Autodesk Inventor part; units mm, degrees
ref_plane "YZ Plane" through (0, 0, 0) normal (1, 0, 0) x (0, 1, 0)
ref_plane "XZ Plane" through (0, 0, 0) normal (0, 1, 0) x (-1, 0, 0)
ref_plane "XY Plane" through (0, 0, 0) normal (0, 0, 1) x (1, 0, 0)
sketch "Sketch1" plane through (0, 0, 0) normal (0, 1, 0) x (-1, 0, 0)
  line L0 (0, 0) -> (-762, 0)
  line L1 (-762, 0) -> (-762, -914.4)
  line L2 (-762, -914.4) -> (0, -914.4)
  line L3 (0, -914.4) -> (0, 0)
  dimension "d0" = 762
  dimension "d1" = 914.4
extrude "Extrusion1" add sketch "Sketch1" along normal blind 19.05
sketch "Sketch5" plane through (762, 0, -914.4) normal (0, 0, -1) x (-1, 0, 0)
  line L0 (0, 0) -> (0, 19.05)
  line L1 (0, 0) -> (762, 0)
  line L2 (762, 0) -> (762, 19.05)
  line L3 (762, 628.65) -> (762, 781.05)
  line L4 (762, 781.05) -> (0, 609.6)
  line L5 (0, 609.6) -> (762, 609.6) construction
  line L6 (762, 19.05) -> (762, 628.65) construction
  line L7 (762, 781.05) -> (757.8183, 799.6354)
  line L8 (757.8183, 799.6354) -> (-4.1817, 628.1854)
  line L9 (0, 609.6) -> (84.6693, 628.65)
  line L10 (-4.1817, 628.1854) -> (0, 609.6)
  line L11 (0, 19.05) -> (762, 19.05)
  dimension "d22" = 152.4
  dimension "d23" = 12.68
  dimension "d25" = 19.05
  dimension "d26" = 90
  dimension "d28" = 90
  dimension "d29" = 90
extrude "Extrusion5" add sketch "Sketch5" against normal up to surface (914.4 mm away) contours L4 L10 L8 L7
sketch "Sketch7" plane through (0, 19.05, 0) normal (0, 1, 0) x (1, 0, 0)
  line L0 (0, 0) -> (762, 0)
  line L1 (0, 914.4) -> (0, 0)
  line L2 (762, 914.4) -> (0, 914.4)
  line L3 (762, 0) -> (762, 914.4)
  line L4 (762, 0) -> (762, 914.4)
  line L5 (0, 914.4) -> (0, 0)
  line L6 (762, 914.4) -> (0, 914.4)
  line L7 (0, 914.4) -> (0, 895.35)
  line L8 (0, 895.35) -> (742.95, 895.35)
  line L9 (762, 895.35) -> (762, 914.4)
  line L10 (762, 914.4) -> (742.95, 914.4)
  line L11 (742.95, 895.35) -> (742.95, 457.2)
  line L12 (742.95, 457.2) -> (762, 457.2)
  line L13 (762, 457.2) -> (762, 914.4)
  dimension "d38" = 19.05
  dimension "d39" = 19.05
  dimension "d40" = 457.2
extrude "Extrusion7" add sketch "Sketch7" along normal blind 609.6 contours L1 L2 L3 L12 L11 L8
sketch "Sketch8" plane through (762, 0, -914.4) normal (0, 0, -1) x (-1, 0, 0)
  line L0 (0, 0) -> (762, 0)
  line L1 (762, 0) -> (762, 628.65)
  line L2 (84.6667, 628.65) -> (762, 628.65)
  line L3 (84.6667, 628.65) -> (762, 781.05)
  line L4 (762, 781.05) -> (757.8183, 799.6354)
  line L5 (757.8183, 799.6354) -> (-4.1817, 628.1854)
  line L6 (-4.1817, 628.1854) -> (0, 609.6)
  line L7 (0, 0) -> (0, 609.6)
  line L8 (762, 628.65) -> (762, 781.05)
  line L9 (84.6667, 628.65) -> (762, 781.05)
  line L10 (762, 781.05) -> (84.6667, 628.65)
  line L11 (84.6667, 628.65) -> (762, 628.65)
extrude "Extrusion8" add sketch "Sketch8" against normal blind 19.05 contours L2 L3 L8
ref_plane "Work Plane2" through (762, 0, -457.2) normal (0, 0, -1) x (-1, 0, 0)
mirror "Mirror1" about plane through (762, 0, -457.2) normal (0, 0, -1) of "Extrusion7"
sketch "Sketch9" plane through (0, 0, 0) normal (0, 0, 1) x (1, 0, 0)
  line L0 (766.1817, 628.1854) -> (762, 609.6)
  line L1 (4.1817, 799.6354) -> (766.1817, 628.1854)
  line L2 (0, 781.05) -> (4.1817, 799.6354)
  line L3 (677.3333, 628.65) -> (0, 781.05)
  line L4 (677.3333, 628.65) -> (0, 628.65)
  line L5 (0, 0) -> (0, 628.65)
  line L6 (0, 0) -> (762, 0)
  line L7 (762, 0) -> (762, 609.6)
  line L8 (0, 19.05) -> (0, 781.05)
  line L9 (0, 628.65) -> (0, 781.05)
  line L10 (0, 781.05) -> (677.3333, 628.65)
  line L11 (0, 781.05) -> (742.95, 613.8863)
  line L12 (0, 628.65) -> (677.3333, 628.65)
extrude "Extrusion9" add sketch "Sketch9" against normal blind 19.05 contours L3 L4 L8
sketch "Sketch12" plane through (742.95, 19.05, -895.35) normal (-1, 0, 0) x (0, 0, 1)
  line L0 (0, 594.8363) -> (876.3, 594.8363)
  line L1 (0, 0) -> (0, 594.8363)
  line L2 (876.3, 0) -> (0, 0)
  line L3 (876.3, 0) -> (876.3, 594.8363)
  line L4 (0, 0) -> (0, 594.8363)
  line L5 (876.3, 0) -> (876.3, 762)
  line L6 (0, 442.4363) -> (876.3, 442.4363)
  line L7 (876.3, 442.4363) -> (876.3, 423.3862)
  line L8 (876.3, 423.3862) -> (0, 423.3862)
  line L9 (0, 423.3862) -> (0, 442.4363)
  point P0 (895.35, -19.05)
  dimension "d57" = 19.05
  dimension "d58" = 152.4
extrude "Extrusion10" add sketch "Sketch12" along normal up to surface (742.95 mm away) contours L6 L3 L8 L1
sketch "Sketch13" plane through (742.95, 461.4863, -19.05) normal (0, 1, 0) x (1, 0, 0)
  line L0 (-742.95, 0) -> (-742.95, 876.3)
  line L1 (0, 876.3) -> (-742.95, 876.3)
  line L2 (0, 0) -> (0, 876.3)
  line L3 (-742.95, 0) -> (0, 0)
  line L4 (0, 0) -> (0, 876.3)
  line L5 (-742.95, 876.3) -> (-742.95, 0)
  line L6 (0, 438.15) -> (-742.95, 438.15)
  line L7 (-742.95, 438.15) -> (-742.95, 419.1)
  line L8 (-742.95, 419.1) -> (0, 419.1)
  line L9 (0, 419.1) -> (0, 438.15)
  point P0 (-742.95, -19.05)
  dimension "d61" = 19.05
extrude "Extrusion11" add sketch "Sketch13" along normal up to surface contours L0 L6 L2 L8 surface through (0, 781.05, -914.4) normal (-0.2195, -0.9756, 0)
sketch "Sketch14" plane through (4.1817, 799.6354, -914.4) normal (-0.9756, 0.2195, 0) x (0, 0, 1)
  line L0 (914.4, -19.05) -> (914.4, 0)
  line L1 (0, 0) -> (914.4, 0)
  line L2 (0, -19.05) -> (0, 0)
  line L3 (0, -19.05) -> (19.05, -19.05)
  line L4 (19.05, -19.05) -> (457.2, -19.05)
  line L5 (457.2, -19.05) -> (476.25, -19.05)
  line L6 (476.25, -19.05) -> (895.35, -19.05)
  line L7 (895.35, -19.05) -> (914.4, -19.05)
  line L8 (914.4, -781.05) -> (914.4, -19.05)
  line L9 (0, 0) -> (914.4, 0)
  line L10 (914.4, 0) -> (914.4, -19.05)
  line L11 (914.4, -19.05) -> (0, -19.05)
  line L12 (0, -19.05) -> (0, 0)
extrude "Extrusion12" add sketch "Sketch14" along normal blind 127
sketch "Sketch15" plane through (742.95, 19.05, -895.35) normal (-1, 0, 0) x (0, 0, 1)
  line L0 (876.3, 423.3862) -> (0, 423.3862)
  line L1 (0, 0) -> (0, 423.3862)
  line L2 (876.3, 0) -> (0, 0)
  line L3 (876.3, 0) -> (876.3, 423.3862)
  line L4 (876.3, 423.3862) -> (0, 423.3862)
  line L5 (0, 0) -> (876.3, 0)
  line L6 (438.15, 423.3862) -> (457.2, 423.3862)
  line L7 (457.2, 423.3862) -> (457.2, 0)
  line L8 (457.2, 0) -> (438.15, 0)
  line L9 (438.15, 0) -> (438.15, 423.3862)
  point P0 (895.35, -19.05)
  dimension "d66" = 19.05
extrude "Extrusion13" add sketch "Sketch15" along normal up to surface (742.95 mm away) contours L7 L2 L9 L0
sketch "Sketch16" plane through (742.95, 19.05, -438.15) normal (0, 0, 1) x (1, 0, 0)
  line L0 (-742.95, 0) -> (-742.95, 423.3862)
  line L1 (0, 423.3862) -> (-742.95, 423.3862)
  line L2 (0, 0) -> (0, 423.3862)
  line L3 (-742.95, 0) -> (0, 0)
  line L4 (0, 0) -> (0, 423.3862)
  line L5 (-742.95, 277.3362) -> (0, 277.3362)
  line L6 (0, 277.3362) -> (0, 296.3862)
  line L7 (0, 296.3862) -> (-742.95, 296.3862)
  line L8 (-742.95, 296.3862) -> (-742.95, 277.3362)
  line L9 (-742.95, 150.3362) -> (0, 150.3362)
  line L10 (0, 150.3362) -> (0, 131.2862)
  line L11 (0, 131.2862) -> (-742.95, 131.2862)
  line L12 (-742.95, 131.2862) -> (-742.95, 150.3362)
  point P0 (-742.95, -19.05)
  dimension "d69" = 19.05
  dimension "d70" = 127
  dimension "d71" = 19.05
  dimension "d72" = 127
extrude "Extrusion14" add sketch "Sketch16" along normal up to surface (419.1 mm away) contours L0 L9 L2 L11 | L0 L7 L2 L5
sketch "Sketch17" plane through (742.95, 19.05, -457.2) normal (0, 0, -1) x (-1, 0, 0)
  line L0 (742.95, 423.3862) -> (0, 423.3862)
  line L1 (0, 0) -> (742.95, 0)
  line L2 (0, 131.2862) -> (0, 0)
  line L3 (0, 277.3362) -> (0, 150.3362)
  line L4 (0, 423.3862) -> (0, 296.3862)
  line L5 (742.95, 423.3862) -> (742.95, 296.3862)
  line L6 (742.95, 277.3362) -> (742.95, 150.3362)
  line L7 (742.95, 131.2862) -> (742.95, 0)
  line L8 (0, 423.3862) -> (742.95, 0) construction
  line L9 (742.95, 423.3862) -> (0, 0) construction
  line L10 (0, 202.1681) -> (742.95, 202.1681)
  line L11 (742.95, 202.1681) -> (742.95, 221.2181)
  line L12 (742.95, 221.2181) -> (0, 221.2181)
  line L13 (0, 221.2181) -> (0, 202.1681)
  line L14 (0, 202.1681) -> (742.95, 221.2181) construction
  line L15 (742.95, 202.1681) -> (0, 221.2181) construction
  point P0 (742.95, -19.05)
  point P1 (371.475, 211.6931)
  dimension "d75" = 19.05
extrude "Extrusion15" add sketch "Sketch17" along normal up to surface (438.15 mm away)
sketch "Sketch18" plane through (0, 0, -914.4) normal (-1, 0, 0) x (0, 0, 1)
  line L0 (476.25, 442.4362) -> (476.25, 315.4362)
  line L1 (19.05, 240.2681) -> (19.05, 442.4362)
  line L2 (457.2, 442.4362) -> (19.05, 442.4362)
  line L3 (457.2, 240.2681) -> (457.2, 442.4362)
  line L4 (457.2, 240.2681) -> (19.05, 240.2681)
  line L5 (476.25, 296.3862) -> (476.25, 169.3862)
  line L6 (476.25, 296.3862) -> (895.35, 296.3862)
  line L7 (895.35, 169.3862) -> (895.35, 296.3862)
  line L8 (476.25, 169.3862) -> (895.35, 169.3862)
  line L9 (476.25, 150.3362) -> (895.35, 150.3362)
  line L10 (895.35, 19.05) -> (895.35, 150.3362)
  line L11 (476.25, 19.05) -> (895.35, 19.05)
  line L12 (476.25, 150.3362) -> (476.25, 19.05)
  line L13 (476.25, 315.4362) -> (895.35, 315.4362)
  line L14 (476.25, 442.4362) -> (476.25, 315.4362)
  line L15 (895.35, 442.4362) -> (476.25, 442.4362)
  line L16 (895.35, 315.4362) -> (895.35, 442.4362)
  line L17 (19.05, 461.4863) -> (19.05, 781.05)
  line L18 (0, 781.05) -> (19.05, 781.05)
  line L19 (0, 0) -> (0, 781.05)
  line L20 (0, 0) -> (914.4, 0)
  line L21 (914.4, 0) -> (914.4, 781.05)
  line L22 (895.35, 781.05) -> (914.4, 781.05)
  line L23 (895.35, 461.4863) -> (895.35, 781.05)
  line L24 (476.25, 461.4863) -> (895.35, 461.4863)
  line L25 (476.25, 461.4863) -> (476.25, 781.05)
  line L26 (457.2, 781.05) -> (476.25, 781.05)
  line L27 (457.2, 461.4863) -> (457.2, 781.05)
  line L28 (19.05, 461.4863) -> (457.2, 461.4863)
  line L29 (457.2, 221.2181) -> (19.05, 221.2181)
  line L30 (457.2, 19.05) -> (457.2, 221.2181)
  line L31 (19.05, 19.05) -> (457.2, 19.05)
  line L32 (19.05, 19.05) -> (19.05, 221.2181)
  line L33 (19.05, 461.4863) -> (19.05, 613.8863)
  line L34 (457.2, 240.2681) -> (457.2, 442.4362)
  line L35 (19.05, 461.4863) -> (457.2, 461.4863)
  line L36 (457.2, 461.4863) -> (457.2, 442.4362)
  line L37 (457.2, 442.4362) -> (19.05, 442.4362)
  line L38 (19.05, 442.4362) -> (19.05, 461.4863)
  line L39 (457.2, 240.2681) -> (19.05, 240.2681)
  line L40 (457.2, 221.2181) -> (19.05, 221.2181)
  line L41 (19.05, 240.2681) -> (457.2, 240.2681)
  line L42 (457.2, 240.2681) -> (457.2, 221.2181)
  line L43 (457.2, 221.2181) -> (19.05, 221.2181)
  line L44 (19.05, 221.2181) -> (19.05, 240.2681)
  line L45 (476.25, 461.4863) -> (476.25, 781.05)
  line L46 (895.35, 315.4362) -> (895.35, 442.4362)
  line L47 (476.25, 461.4863) -> (895.35, 461.4863)
  line L48 (895.35, 461.4863) -> (895.35, 442.4362)
  line L49 (895.35, 442.4362) -> (476.25, 442.4362)
  line L50 (476.25, 442.4362) -> (476.25, 461.4863)
  line L51 (895.35, 169.3862) -> (895.35, 296.3862)
  line L52 (476.25, 315.4362) -> (895.35, 315.4362)
  line L53 (895.35, 315.4362) -> (895.35, 296.3862)
  line L54 (895.35, 296.3862) -> (476.25, 296.3862)
  line L55 (476.25, 296.3862) -> (476.25, 315.4362)
  line L56 (476.25, 169.3862) -> (895.35, 169.3862)
  line L57 (895.35, 19.05) -> (895.35, 150.3362)
  line L58 (476.25, 169.3862) -> (895.35, 169.3862)
  line L59 (895.35, 169.3862) -> (895.35, 150.3362)
  line L60 (895.35, 150.3362) -> (476.25, 150.3362)
  line L61 (476.25, 150.3362) -> (476.25, 169.3862)
extrude "Extrusion16" cut sketch "Sketch18" against normal blind 12.7 contours L50 L24 L48 L15 | L13 L53 L6 L55 | L8 L59 L9 L61 | L36 L2 L38 L28 | L42 L29 L44 L4
properties part number "Top"
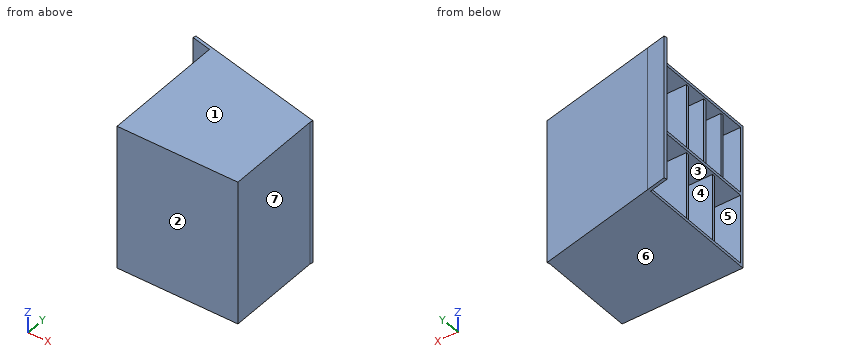
Source: CAD feature listing. Evaluate the final solid. Frame: model axes, mm. Face numbers are marked on the shaded views. A direction names the side the tool comes from. Give positions to 0.01 mm unless a question says otherwise; leave off trailing zeros. Loops run counter-clockwise (first coordinate to the right, second up) from the corner with the lowest first, then second, coordinate; pieces in that order, holes last. Notation, with made-up numbers: (61, 63) - (103, 63) arc R16 ccw to (103, 79) - close; hole circle Ø6 at (74.25, 86). An arc over 180 degrees is marked (long way). Use CSV: the item, a comma, the result in double quotes.
1) Line query: line 1 (Z direction, x = 90.5, y = 629); line 2 (Y direction, x = 43, z = -859.5) (3 decimals); line 3 (Y direction, x = 442.5, z = -286.5). Output: solid intervals per line, ascending.
Worked out:
line 1,"z = -914.4 to -895.35, -457.2 to -438.15, -19.05 to 0"
line 2,"y = 0 to 19.05, 221.218 to 240.268, 442.436 to 461.486, 771.375 to 790.901"
line 3,"y = 0 to 19.05, 150.34 to 169.39, 296.39 to 315.44, 442.44 to 461.49, 681.49 to 701.01"
2) Cut plane C-C (y = 109.5). Output: boundary loops of the cut face in (x, z).
Worked out:
outline,"(0, -914.4) - (762, -914.4) - (762, 0) - (0, 0) - (0, -19.05) - (742.95, -19.05) - (742.95, -438.15) - (0, -438.15) - (0, -457.2) - (742.95, -457.2) - (742.95, -895.35) - (0, -895.35) - close"
3) Mould query, pull axis Y, two halves, no side actions, for the marked faces 1, 2, 3 and 4. Classes: +Y half, -Y half, draft (parallel to the pull), parting line (faces both ways), or undercut.
Worked out:
face 1,"draft"
face 2,"-Y half"
face 3,"undercut"
face 4,"undercut"
4) Set-up query: the marked faces 5, 6 and 7. Return all of +Z, -Z, +X, -X, +Y, -Y with unobstructed straight access to the full face (end or side cutting, diameter ignored); none if empty.
Worked out:
face 5,"-X"
face 6,"-Z, +X, -X, +Y, -Y"
face 7,"+Z, -Z, +X, -Y"
5) Pin query (flat end, axial travel): P1, Ø9.5, axis at y = 230, z = -675, coming from the -X side; P2, Ø4, axis at x = 556.5, z = -638, coming from the +Y side; P3, Ø1, axis at x = 526, z = -99.5, coming from the +Y side. Return the tip coordinate at first contact, or that it passes through.
Worked out:
P1,"stops at x = 12.7"
P2,"stops at y = 675.81"
P3,"stops at y = 682.34"
6) Cut plane A-A (x = 269.5). Count the separate pieces of the cut face and the enclosed holes in it, and give its area (3 significant figures).
Worked out:
separate pieces,"1"
enclosed holes,"7"
area,"116,000 mm^2"
7) Cut plane B-B (z = -750.5). Output: boundary loops of the cut face in (x, y), and give its area (3 significant figures).
Worked out:
outline,"(-123.9, 808.93) - (0, 781.05) - (742.95, 613.89) - (742.95, 461.49) - (12.7, 461.49) - (12.7, 442.44) - (742.95, 442.44) - (742.95, 240.27) - (12.7, 240.27) - (12.7, 221.22) - (742.95, 221.22) - (742.95, 19.05) - (0, 19.05) - (0, 0) - (762, 0) - (762, 609.6) - (766.18, 628.19) - (4.18, 799.64) - (-119.72, 827.51) - close"
area,"70,900 mm^2"
